Verification items for this drawing (mm, ordinates from the low corner). A direction names the side the tool comes from. Coordinates: 2 decimals unless noted, no trailing zeros. Write each loop counter-clockwise with the first axis right and the second up, starting at its lowest first coordinate (ties: lowest second). Pieces come first, ordered by that corner, then holes. Notation, with made-up numbers: M 86.25,26 L 145.25,26 A14 cw 145.25,40 Z; hole C -31,-30.5 d3. An arc over 180 degrees is marked long. Answer as CSV lines item,"result". Start each with the question number.
1) Go/stop test with flat-tipped pins: pin 1 Ø6 at (x, z) = (24.5, 66) entering from -Y; pin 2 Ø5 at (y, z) = (11.5, 94.43) entering from -X; pin 3 Ø8 at (y, z) = (11.5, 33) entering from -X; pin 4 Ø1.5 at (x, y) = (54.5, 11) entering from -Z. Record where each tip stops, or that it passes through.
2) Access from +Z, -Z, +X, -X, +Y, -Y to the whole of each face (thin tool, end or side, straight path). Record for the marked faces 1 and 2.
3) Section check B-B (y = 11.5). Record the cut outline in (x, z).
4) Material ranges on L1, parallel to X at y = 16.75, z = 93.5; L2, parallel to Y at x = 46.4, z = 82.46; L3, parallel to Y at x = 47.5, z = 5.5, recorded low to high. Write a range as [from, to].
5) Section check C-C (x = 24.5). Record the cut outline in (y, z).
6) Section check D-D (z = 49.5). Record the cut outline in (x, y), and give its area (3 significant figures).
7) Section check A-A (z = 82.46). Record the cut outline in (x, y), and give its area (3 significant figures).
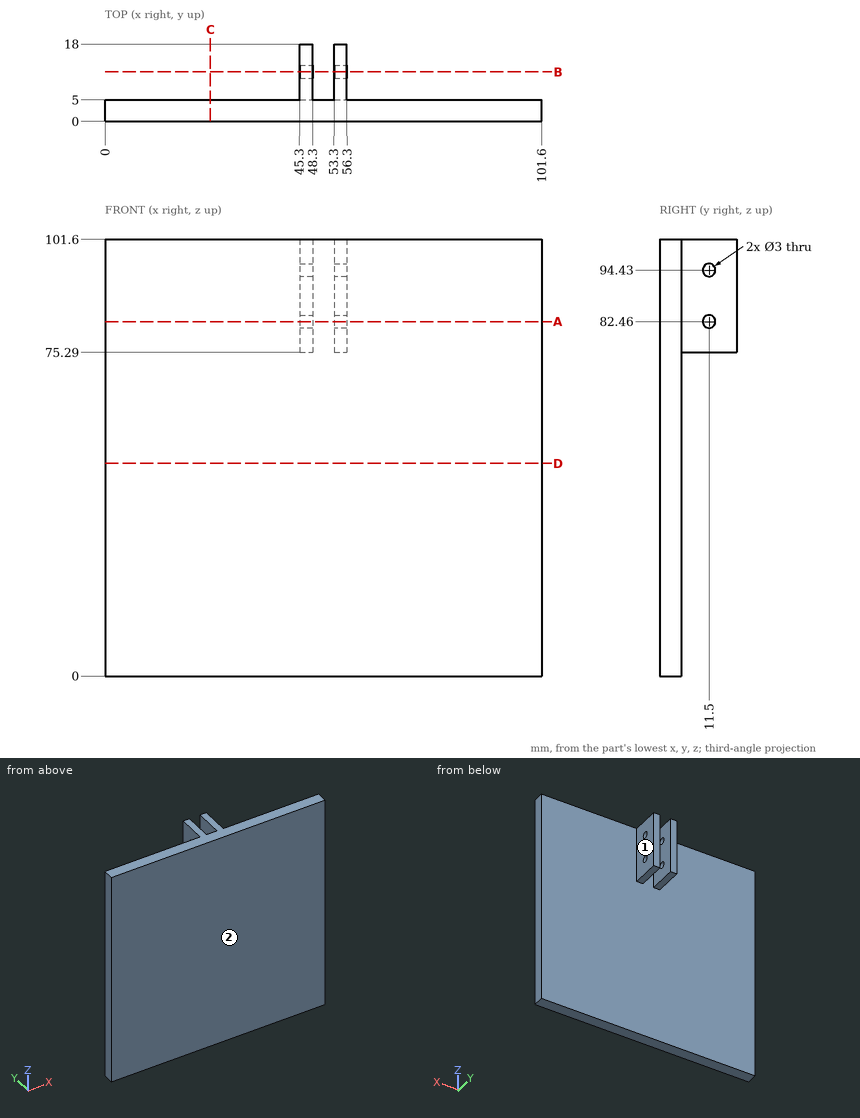
Results found:
1,pin 1,"stops at y = 0"
1,pin 2,"stops at x = 45.3"
1,pin 3,"passes through"
1,pin 4,"stops at z = 75.29"
2,face 1,"+Z, -Z, +X, +Y"
2,face 2,"+Z, -Z, +X, -X, -Y"
3,outline,"M 45.3,75.29 L 48.3,75.29 L 48.3,80.96 L 45.3,80.96 Z; M 45.3,83.96 L 48.3,83.96 L 48.3,92.93 L 45.3,92.93 Z; M 45.3,95.93 L 48.3,95.93 L 48.3,101.6 L 45.3,101.6 Z; M 53.3,75.29 L 56.3,75.29 L 56.3,80.96 L 53.3,80.96 Z; M 53.3,83.96 L 56.3,83.96 L 56.3,92.93 L 53.3,92.93 Z; M 53.3,95.93 L 56.3,95.93 L 56.3,101.6 L 53.3,101.6 Z"
4,L1,"x = [45.3, 48.3], [53.3, 56.3]"
4,L2,"y = [0, 10], [13, 18]"
4,L3,"y = [0, 5]"
5,outline,"M 0,0 L 5,0 L 5,101.6 L 0,101.6 Z"
6,outline,"M 0,0 L 101.6,0 L 101.6,5 L 0,5 Z"
6,area,"508 mm2"
7,outline,"M 0,0 L 101.6,0 L 101.6,5 L 56.3,5 L 56.3,10 L 53.3,10 L 53.3,5 L 48.3,5 L 48.3,10 L 45.3,10 L 45.3,5 L 0,5 Z; M 45.3,13 L 48.3,13 L 48.3,18 L 45.3,18 Z; M 53.3,13 L 56.3,13 L 56.3,18 L 53.3,18 Z"
7,area,"568 mm2"
